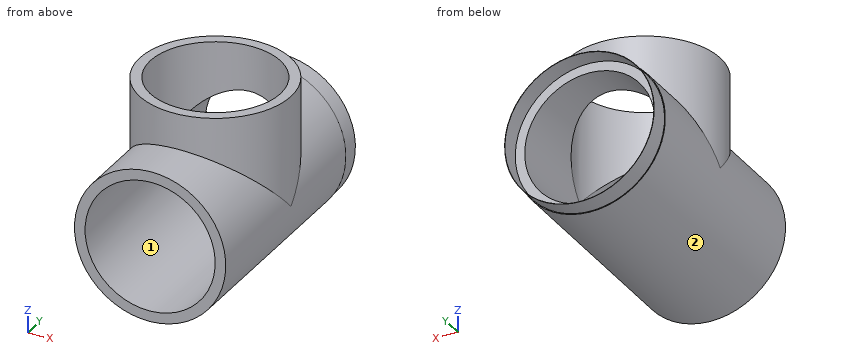
from build123d import *

# Parameters (mm, degrees)
SKETCH_1_R          = 232.5
SKETCH_1_R_2        = 200
EXTRUDE_1_DEPTH     = 698
SKETCH_11_R         = 230
SKETCH_11_R_2       = 229
EXTRUDE_1_2_DEPTH   = 60
SKETCH_12_R         = 232.5
SKETCH_12_R_2       = 200
EXTRUDE_2_DEPTH     = 341
SKETCH_13_R         = 200
CUT_EXTRUDE_1_DEPTH = 380
CUT_EXTRUDE_START   = -1000
SKETCH_14_R         = 200
CUT_EXTRUDE_2_DEPTH = 1000


with BuildPart() as part:
    # Эскиз1 → Extrude 1 (new body)
    with BuildSketch(Plane(origin=(0, 0, 0), x_dir=(1, 0, 0), z_dir=(0, 1, 0))):
        with Locations(Location((0, 0, 0), (0, 0, 270))):
            Circle(SKETCH_1_R)
        with Locations(Location((0, 0, 0), (0, 0, 270))):
            Circle(SKETCH_1_R_2, mode=Mode.SUBTRACT)
    extrude(amount=EXTRUDE_1_DEPTH)

    # Эскиз11 → Extrude 1 2 (add)
    with BuildSketch(Plane(origin=(0, 698, 0), x_dir=(1, 0, 0), z_dir=(0, 1, 0))):
        with Locations(Location((0, 0, 0), (0, 0, 270))):
            Circle(SKETCH_11_R)
        with Locations(Location((0, 0, 0), (0, 0, 270))):
            Circle(SKETCH_11_R_2, mode=Mode.SUBTRACT)
    extrude(amount=EXTRUDE_1_2_DEPTH)

    # Эскиз12 → Бобышка-Вытянуть2 (add)
    with BuildSketch(Plane.XY):
        with Locations((0, 379)):
            Circle(SKETCH_12_R)
        with Locations(Location((0, 379, 0), (0, 0, 180))):
            Circle(SKETCH_12_R_2, mode=Mode.SUBTRACT)
    extrude(amount=EXTRUDE_2_DEPTH)

    # Эскиз13 → Вырез-Вытянуть1 (cut)
    with BuildSketch(Plane.XY):
        with Locations((0, 379)):
            Circle(SKETCH_13_R)
    extrude(amount=CUT_EXTRUDE_1_DEPTH, mode=Mode.SUBTRACT)

    # Эскиз14 → Вырез-Вытянуть2 (cut)
    with BuildSketch(Plane(origin=(0, 698, 0), x_dir=(1, 0, 0), z_dir=(0, 1, 0)).offset(CUT_EXTRUDE_START)):
        with Locations(Location((0, 0, 0), (0, 0, 270))):
            Circle(SKETCH_14_R)
    extrude(amount=CUT_EXTRUDE_2_DEPTH, mode=Mode.SUBTRACT)


solid = part.part
Geometry: final body of the model. Coordinates: model frame, mm. Face numbers are marked on the shaded views. Give positions to 0.01 mm unless a question says otherwise; leave off trailing zeros. Write each loop counter-clockwise with the first axis right and the second up, starting at its lowest first coordinate (ties: lowest second). Pieces come first, ordered by that corner, then holes. Notation, with made-up numbers: (71, 86) -> (110, 86) arc R18 ccw to (110, 106) -> close; hole circle Ø4 at (-1, -34). An arc over 180 degrees is marked (long way). Answer as a JSON object with one key per item and string values.
1. Contact query for flat-ended pins moving along their axis: pin 1 (12 mm diameter, centred on y = 462, z = -64, fed in from -X); pin 2 (8 mm diameter, centred on x = 184.5, y = 179.5, fed in from -Z); pin 3 (5 mm diameter, centred on y = 364, z = -136, fed in from -X). Output: stop coordinate, or through.
Ans:
{"pin 1": "stops at x = -225.15", "pin 2": "stops at z = -146.55", "pin 3": "stops at x = -190.35"}
2. Cut plane B-B on y = 324.5. Output: boundary loops of the cut face in (x, z).
Ans:
{"outline": "(-226.02, 54.5) arc R232.5 ccw (long way) to (226.02, 54.5) -> (226.02, 341) -> (192.43, 341) -> (192.43, 54.5) arc R200 cw (long way) to (-192.43, 54.5) -> (-192.43, 341) -> (-226.02, 341) -> close"}
3. Ray query, probe 1 along X at (y, z) = (516, 0); probe 2 along Y at (x, z) = (0, 244); probe 3 along X at (y, z) = (738, 0). Return the intervals inside material, ascending. Write a range as from..to.
Ans:
{"probe 1": "x = -232.5..-200, 200..232.5", "probe 2": "y = 146.5..179, 579..611.5", "probe 3": "x = -230..-229, 229..230"}
4. Mould query, pull axis Z, two halves, no side actions, for the marked faces 1 and 2. Classes: pulls with the +Z half, pulls with the -Z half, needs draft (parallel to the pull), parting line crosses it, or undercut.
Ans:
{"face 1": "undercut", "face 2": "parting line crosses it"}
5. Cut plane D-D on z = 273. Output: boundary loops of the cut face in (x, y).
Ans:
{"outline": "circle Ø465 at (0, 379); hole circle Ø400 at (0, 379)"}
6. Cut plane C-C on z = -24.5. Output: boundary loops of the cut face in (x, y).
Ans:
{"outline": "(-231.21, 0) -> (-198.49, 0) -> (-198.49, 698) -> (-227.69, 698) -> (-227.69, 758) -> (-228.69, 758) -> (-228.69, 698) -> (-231.21, 698) -> close; (198.49, 0) -> (231.21, 0) -> (231.21, 698) -> (228.69, 698) -> (228.69, 758) -> (227.69, 758) -> (227.69, 698) -> (198.49, 698) -> close"}
